Verification items for the finished model (mm, model axes). Face numbers are marked on the shaded views. A direction names the side the tool comes from. Give positions to 0.01 mm unless a question says otherwise; leave off trailing zeros. Write each loop counter-clockwise with the first axis right and the second up, starting at its lowest first coordinate (ties: lowest second). Pieces come first, ordered by that corner, then holes. Notation, with made-up numbers: (-33, 33) - (-17, 33) arc R10 cw to (-17, 45) - close; hole circle Ø10 at (67, 26). An arc over 180 degrees is marked (long way). Answer as a JSON object with one key per item and string values. Group by question number.
Item 1: Sectioned sample at A-A, the plane z = 0. Record the boundary of the cut face in (x, y) (3 decimals).
Item 2: Sectioned sample at B-B, the plane x = 0. Record the boundary of the cut face in (y, z) (3 decimals), and give its area (3 significant figures).
Item 3: Sectioned sample at C-C, the plane y = 17.5. Record the boundary of the cut face in (x, z).
Item 4: Sectioned sample at D-D, the plane x = -2.25. Record the boundary of the cut face in (y, z), and give its area (3 significant figures).
Item 5: Go/stop test with flat-tipped pins: pin 1 (3 mm diameter, centred on x = -1.5, z = -1, fed in from +Y); pin 2 (8 mm diameter, centred on y = 15, z = 5, fed in from +X); pin 3 (4 mm diameter, centred on x = -5.5, y = 3, fed in from +Z); pin 4 (3 mm diameter, centred on x = 0.5, z = 1, fed in from -Y). Record where each tip stops, or that it passes through.
Item 6: Tool access check on the marked faces 4 and 5. Record the directions out of +Z, -Z, +X, -X, +Y, -Y that give a thin tool (end or side, any length) a straight path to the whole face; none if there is none.
Item 7: Scan lines: line 1 along Z through (x, y) = (0, 7.5) (3 decimals); line 2 along Z through (x, y) = (-0.25, 22.5); line 3 along X through (y, z) = (4, -2.5). Record each from-to range of solid material in increasing order. Write a range as [from, to].
Item 8: Draft check along Z on the marked faces 1, 2 and 3. Enter one of: +Z half, -Z half, draft (parallel to the pull), parting line (faces both ways), or undercut.
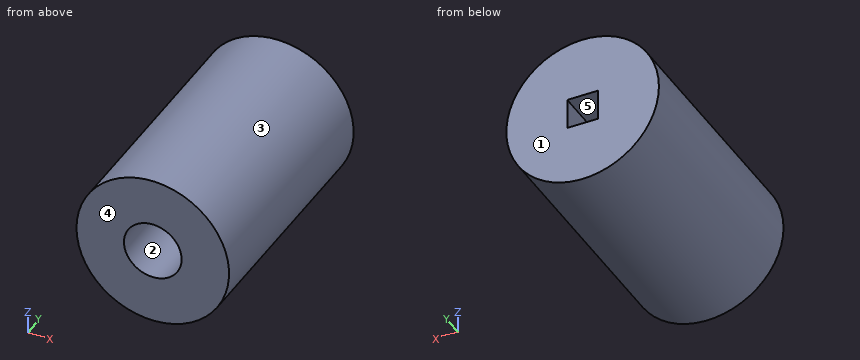
Autodesk Inventor part; units mm, degrees
ref_plane "YZ Plane" through (0, 0, 0) normal (1, 0, 0) x (0, 1, 0)
ref_plane "XZ Plane" through (0, 0, 0) normal (0, 1, 0) x (-1, 0, 0)
ref_plane "XY Plane" through (0, 0, 0) normal (0, 0, 1) x (1, 0, 0)
sketch "Sketch1" plane through (0, 0, 0) normal (0, 1, 0) x (-1, 0, 0)
  circle A0 centre (0, 0) radius 8
  dimension "d0" = 16
extrude "Extrusion1" add sketch "Sketch1" along normal blind 25.4
sketch "Sketch3" plane through (0, 25.4, 0) normal (0, 1, 0) x (1, 0, 0)
  line L0 (-1.61, -1.61) -> (1.61, -1.61)
  line L1 (1.61, -1.61) -> (1.61, 1.61)
  line L2 (1.61, 1.61) -> (-1.61, 1.61)
  line L3 (-1.61, 1.61) -> (-1.61, -1.61)
  point P0 (0, 0)
  dimension "d13" = 3.22
  dimension "d15" = 1.61
  dimension "d16" = 1.61
extrude "Extrusion2" cut sketch "Sketch3" against normal blind 12.7
sketch "Sketch4" plane through (0, 0, 0) normal (0, -1, 0) x (1, 0, 0)
  circle A0 centre (0, 0) radius 3.025
  dimension "d19" = 6.05
extrude "Extrusion3" cut sketch "Sketch4" against normal blind 12.7
properties part number "Wheel_Coupler"
Geometry check:
{
 "1": {"outline": "(-8, 0) - (-3.025, 0) - (-3.025, 12.7) - (-1.61, 12.7) - (-1.61, 25.4) - (-8, 25.4) - close; (1.61, 12.7) - (3.025, 12.7) - (3.025, 0) - (8, 0) - (8, 25.4) - (1.61, 25.4) - close"},
 "2": {"outline": "(0, -8) - (25.4, -8) - (25.4, -1.61) - (12.7, -1.61) - (12.7, -3.025) - (0, -3.025) - close; (0, 3.025) - (12.7, 3.025) - (12.7, 1.61) - (25.4, 1.61) - (25.4, 8) - (0, 8) - close", "area": "289 mm^2"},
 "3": {"outline": "circle Ø16 at (0, 0); hole (-1.61, -1.61) - (1.61, -1.61) - (1.61, 1.61) - (-1.61, 1.61) - close"},
 "4": {"outline": "(0, -7.68) - (25.4, -7.68) - (25.4, 7.68) - (0, 7.68) - (0, 2.02) - (12.7, 2.02) - (12.7, -2.02) - (0, -2.02) - close", "area": "339 mm^2"},
 "5": {"pin 1": "y = 25.4", "pin 2": "x = 7.94", "pin 3": "z = 7.19", "pin 4": "y = 12.7"},
 "6": {"face 4": "+Z, -Z, +X, -X, -Y", "face 5": "+Y, -Y"},
 "7": {"line 1": "[-8, -3.025], [3.025, 8]", "line 2": "[-8, -1.61], [1.61, 8]", "line 3": "[-7.6, -1.7], [1.7, 7.6]"},
 "8": {"face 1": "draft", "face 2": "undercut", "face 3": "parting line"}
}
